CAD build for the part. Positions are in the model's coordinates, mm. Face numbers are marked on the shaded views. A direction names the side the tool comes from. Round coordinates to 2 decimals unless told otherwise and drop trailing zeros. Write each loop counter-clockwise with the first axis right and the second up, starting at its lowest first coordinate (ties: lowest second). Pieces come first, ordered by that corner, then holes. Notation, with made-up numbers: (44, 66) - (80, 66) arc R14 cw to (80, 92) - close; hole circle Ø7 at (28, 18.25). An arc over 180 degrees is marked (long way). Use one line per item in the form item = value. Start each with the question number.
Item 1: Band-saw the part on C-C, the plane y = 28.5. List the corners of the cut face in (x, z).
Item 2: Pull direction X, two halves, no side cores. Call the marked faces 4, 5, 6 and 7: +X half, -X half, draft (parallel to the pull), parting line (faces both ways), or undercut.
Item 3: Band-saw the part on A-A, the plane z = 0. List the corners of the cut face in (x, y), and give its area (3 significant figures).
Item 4: Band-saw the part on B-B, the plane x = -13. List the corners of the cut face in (y, z).
Item 5: Pin check, flat tips, straight feed: pin 1 (1.5 mm diameter, centred on x = 6.5, z = 25.5, fed in from -Y); pin 2 (1 mm diameter, centred on y = 61.5, z = -3, fed in from -X); pin 3 (10 mm diameter, centred on y = 9.5, z = -22, fed in from +X). Stop position of each tip, or through.
Item 6: Band-saw the part on D-D, the plane y = 46. List the corners of the cut face in (x, z), and give its area (3 significant figures).
Item 7: Tool access for the marked faces 1, 2 and 3: list every direction of +Z, -Z, +X, -X, +Y, -Y with a clear straight run to the whole face (end or side of a thin tool).
Item 8: Drill centre lines: L1, parallel to Y at x = 29.5, z = 36.5; L2, parallel to Y at x = -15, z = -3; L3, parallel to X at y = 28, z = -36. Where is each one in solid material? Low to high.
from build123d import *

# Parameters (mm, degrees)
SKETCH_1_R               = 50
EXTRUDE_1_DEPTH          = 100
CUT_EXTRUDE_1_DEPTH      = 123.474487139
CUT_EXTRUDE_1_DEPTH_BACK = 123.474487139


with BuildPart() as part:
    # 草图1 → 凸台-拉伸1 (new body)
    with BuildSketch(Plane(origin=(0, 0, 0), x_dir=(1, 0, 0), z_dir=(0, 1, 0))):
        with Locations(Location((0, 0, 0), (0, 0, 270))):
            Circle(SKETCH_1_R)
    extrude(amount=EXTRUDE_1_DEPTH)

    # 草图2 → 切除-拉伸1 (cut, two sides: drawn at the far end of the back side and taken through both)
    with BuildSketch(Plane.XY.offset(-CUT_EXTRUDE_1_DEPTH_BACK)):
        Polygon((0, 0), (0, 20), (-17.67766953, 2.32233047), (-31.819805153, 16.464466094), (-38.890872965, 9.393398282), (-45.961940777, 16.464466094), (-31.843330798, 30.583076073), (-17.701195174, 16.440940449), (0, 34.142135624), (0, 54.142135624), (63.983037585, 54.142135624), (63.983037585, 0), align=None)
    extrude(amount=CUT_EXTRUDE_1_DEPTH + CUT_EXTRUDE_1_DEPTH_BACK, mode=Mode.SUBTRACT)


solid = part.part
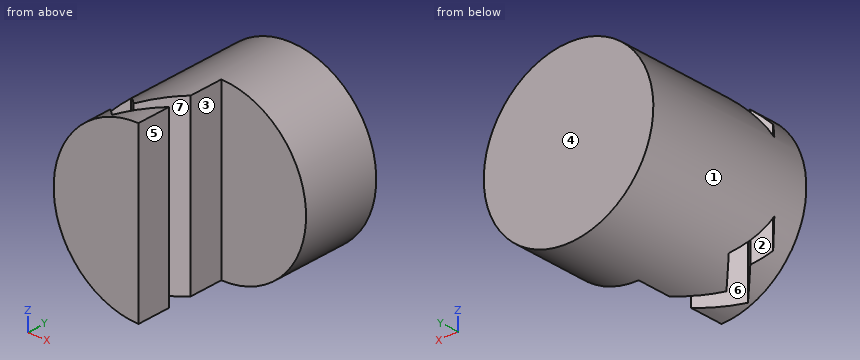
Determined:
q1.outline = (-33.93, -36.73) - (-33.93, 36.73) arc R50 ccw to start; (-29.76, -40.18) arc R50 ccw to (-5.64, -49.68) - (-5.64, 49.68) arc R50 ccw to (-29.76, 40.18) - close
q2.face_4 = draft
q2.face_5 = +X half
q2.face_6 = undercut
q2.face_7 = undercut
q3.outline = (-50, 0) - (0, 0) - (0, 20) - (-17.68, 2.32) - (-31.82, 16.46) - (-38.89, 9.39) - (-45.96, 16.46) - (-31.84, 30.58) - (-17.7, 16.44) - (0, 34.14) - (0, 54.14) - (50, 54.14) - (50, 100) - (-50, 100) - close
q3.area = 6,690 mm²
q4.outline = (0, -48.28) - (7, -48.28) - (7, 48.28) - (0, 48.28) - close; (21.14, -48.28) - (100, -48.28) - (100, 48.28) - (21.14, 48.28) - close
q5.pin_1 = 54.14
q5.pin_2 = -49.94
q5.pin_3 = 0
q6.outline = (0, -50) - (0, 50) arc R50 ccw to start
q6.area = 3,930 mm²
q7.face_1 = +Y, -Y
q7.face_2 = +Z, -Z
q7.face_3 = +Z, -Z, +X, -Y
q8.L1 = 54.14 to 100
q8.L2 = 0 to 5, 19.14 to 100
q8.L3 = -34.7 to -34.43, -29.26 to -6.14
